Input: part model. Units: mm. Frame: model coordinates. Give positions to 0.01 mm unless a question says otherwise; leave off trailing zeros. Loops run counter-clockwise (first coordinate to the right, second up) from the corner with the lowest first, then second, coordinate; pieces in that order, holes last. Notation, with made-up numbers: M 2,1.5 L 44,1.5 A16 ccw 44,23.5 Z; hole C -26,-10 d6. An arc over 180 degrees is marked long. Answer as a JSON object with one key per item and string values. Group by question number.
1) Section query D-D on x = 16. Return loops of the section in (y, z) (3 decimals).
2) Draft query along X for faces 1 (the cylindrical face through (1.096, 2.107, 1.479)), 2 (the flat face through (7, 0, 3)), 3 (the flat face through (8.48, 3.72, 1.48)), 4 (the cylindrical face through (15.076, -0.041, 1.479)). Return one class per face: +X half, -X half, draft (parallel to the pull), parting line (faces both ways), or undercut.
3) Ray query, L1, parallel to Y at x = 16, z = 1.65 (3 decimals); L2, parallel to X at y = 1.5, z = 0.3; L3, parallel to X at y = -1, z = 2.65. Return the intervals inside material, ascending.
4) Section query C-C on z = 0.45. Return loops of the section in (x, y) (3 decimals).
5) Section query A-A on x = 0. Return loops of the section in (y, z) (3 decimals), plus the area to 4 significant figures.
6) First-contact query: P1, Ø3, axis at x = 0, y = 0, coming from the -Z side. Flat tip, straight axial feed; report the tip coordinate or a pass-through.
7) Section query B-B on y = 0. Return loops of the section in (x, z) (3 decimals), plus the area to 3 significant figures.
Autodesk Inventor part; units mm, degrees
ref_plane "YZ Plane" through (0, 0, 0) normal (1, 0, 0) x (0, 1, 0)
ref_plane "XZ Plane" through (0, 0, 0) normal (0, 1, 0) x (-1, 0, 0)
ref_plane "XY Plane" through (0, 0, 0) normal (0, 0, 1) x (1, 0, 0)
sketch "Sketch1" plane through (0, 0, 0) normal (0, 0, 1) x (1, 0, 0)
  circle A0 centre (0, 0) radius 2.375
  line L0 (0.7812, 4.9386) -> (16.3906, 2.4693)
  arc A1 (16.3906, -2.4693) -> (16.3906, 2.4693) centre (16, 0) ccw
  line L1 (16.3906, -2.4693) -> (0.7812, -4.9386)
  arc A2 (0.7812, 4.9386) -> (0.7812, -4.9386) centre (0, 0) ccw
  circle A3 centre (16, 0) radius 0.925
  dimension "d0" = 4.75
  dimension "d3" = 2.5
  dimension "d6" = 5
  dimension "d7" = 16
  dimension "d8" = 1.85
extrude "Extrusion1" add sketch "Sketch1" along normal blind 3
properties part number "slider_link_p2"
Output:
{
 "1": {"outline": "M -2.531,0 L -0.925,0 L -0.925,3 L -2.531,3 Z; M 0.925,0 L 2.531,0 L 2.531,3 L 0.925,3 Z"},
 "2": {"face 1": "undercut", "face 2": "draft", "face 3": "+X half", "face 4": "undercut"},
 "3": {"L1": "y = -2.531 to -0.925, 0.925 to 2.531", "L2": "x = -4.77 to -1.84, 1.84 to 18", "L3": "x = -4.9 to -2.15, 2.15 to 18.29"},
 "4": {"outline": "M 0.781,-4.939 L 16.391,-2.469 A2.5 ccw 16.391,2.469 L 0.781,4.939 A5 ccw long Z; hole C 0,0 d4.75; hole C 16,0 d1.85"},
 "5": {"outline": "M -5,0 L -2.375,0 L -2.375,3 L -5,3 Z; M 2.375,0 L 5,0 L 5,3 L 2.375,3 Z", "area": "15.75 mm^2"},
 "6": {"P1": "passes through"},
 "7": {"outline": "M -5,0 L -2.375,0 L -2.375,3 L -5,3 Z; M 2.375,0 L 15.075,0 L 15.075,3 L 2.375,3 Z; M 16.925,0 L 18.5,0 L 18.5,3 L 16.925,3 Z", "area": "50.7 mm^2"}
}
